Could you check a few things on this drawing? It's one solid part, dimensions in mm from its lowest x, y, z. A direction names the side the tool comes from. Coordinates: 2 decimals unless noted, no trailing zeros. Order: outer loops, then holes, each group sorted by start corner. A loop starts at its lowest first (then second) coordinate and runs counter-clockwise, first axis right, second up. Notation, with made-up numbers: (35, 45.25) - (49, 45.25) arc R25 cw to (49, 82.25) - close; hole circle Ø3 at (33.25, -39). An arc over 180 degrees is marked (long way). Return JSON: item names as keys, results as strings. Group by question number.
1) Imagine slicing it at A-A (z = 10.5). Write out the boundary of the cut face in (x, y).
2) Imagine slicing it at B-B (x = 10.5). Write out the boundary of the cut face in (y, z).
3) Which directions (+Z, -Z, +X, -X, +Y, -Y) give clear straight access to the entire face, cutting with the end or side of a thin tool? Please do the marked faces 1, 2 and 3.
4) Imagine slicing it at D-D (z = 4.25). Write out the boundary of the cut face in (x, y), and give its area (3 significant figures).
5) For pin 1 Ø6 at (x, y) = (13, 10) entering from -Z; pin 2 Ø1.5 at (x, y) = (14, 35) entering from -Z; pin 3 Ø10 at (y, z) = (5.5, 10.5) entering from +X; pin 4 Ø1 at (x, z) = (19, 14.5) entering from -Y, each with a flat end and sliding along its axis, tell me the tip position at first contact or that it passes through.
6) Imagine slicing it at C-C (y = 19). Write out the boundary of the cut face in (x, z).
7) If I drill on line 1 along Z through (x, y) = (10.5, 5.25); line 2 along X through (y, z) = (8, 10.5); line 3 along Z through (x, y) = (10.5, 27), over which ranges is the centre line in solid material (lowest first)?
8) If we mould it in two halves opening along Z, with no side actions, what happens to the marked faces 4, 5 and 6? For each: pulls with the +Z half, pulls with the -Z half, needs draft (parallel to the pull), parting line crosses it, or undercut.
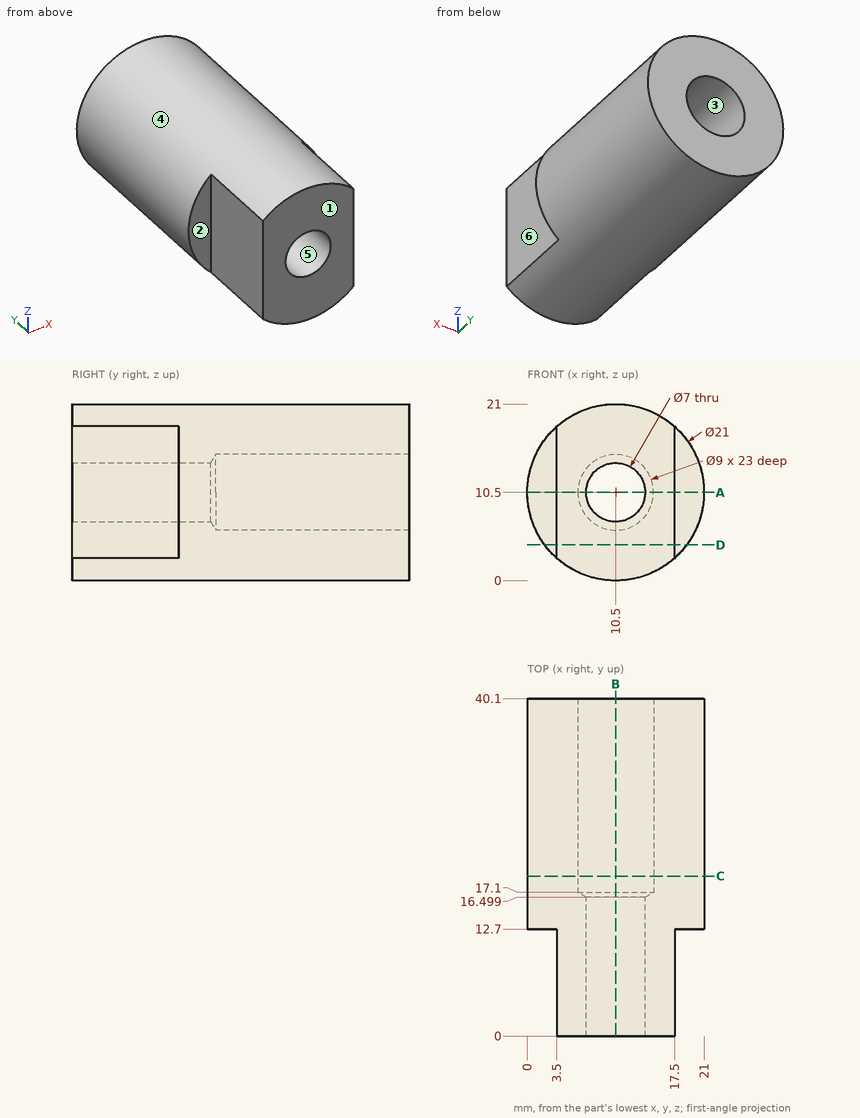
Calculated:
{
 "1": {"outline": "(0, 12.7) - (3.5, 12.7) - (3.5, 0) - (7, 0) - (7, 16.5) - (6, 17.1) - (6, 40.1) - (0, 40.1) - close; (14, 0) - (17.5, 0) - (17.5, 12.7) - (21, 12.7) - (21, 40.1) - (15, 40.1) - (15, 17.1) - (14, 16.5) - close"},
 "2": {"outline": "(0, 0) - (40.1, 0) - (40.1, 6) - (17.1, 6) - (16.5, 7) - (0, 7) - close; (0, 14) - (16.5, 14) - (17.1, 15) - (40.1, 15) - (40.1, 21) - (0, 21) - close"},
 "3": {"face 1": "+Z, -Z, +X, -X, -Y", "face 2": "+Z, -Z, -X, -Y", "face 3": "+Y"},
 "4": {"outline": "(2.06, 12.7) - (3.5, 12.7) - (3.5, 0) - (17.5, 0) - (17.5, 12.7) - (18.94, 12.7) - (18.94, 40.1) - (2.06, 40.1) - close", "area": "640 mm2"},
 "5": {"pin 1": "z = 0", "pin 2": "z = 0.37", "pin 3": "x = 17.5", "pin 4": "y = 12.7"},
 "6": {"outline": "circle Ø21 at (10.5, 10.5); hole circle Ø9 at (10.5, 10.5)"},
 "7": {"line 1": "0 to 7, 14 to 21", "line 2": "3.5 to 7, 14 to 17.5", "line 3": "0 to 6, 15 to 21"},
 "8": {"face 4": "parting line crosses it", "face 5": "undercut", "face 6": "needs draft"}
}
